The drawing under review shows one solid part. Ordinate dimensions are in mm from its lowest x, y, z. A direction names the side the tool comes from. Round coordinates to 2 decimals unless told otherwise and drop trailing zeros. Write each loop counter-clockwise with the first axis right and the second up, starting at its lowest first coordinate (ties: lowest second). Pieces come first, ordered by that corner, then holes.
Item 1: Add section A-A (z = 33). Give the boundary of the cut face in (x, y).
Item 2: Machinability: for the marked faces 1 and 2, which of the approach directions +Z, -Z, +X, -X, +Y, -Y give a long, thin tool a straight path to every point of the face, cutting with its end or side? Answer none if there is none.
Item 3: Add section C-C (x = 36.25). Give the boundary of the cut face in (y, z), plus the area to 3 significant figures.
Item 4: Clearance check with flat-ended pins moving along their axes: pin 1 Ø12 at (x, z) = (26, 10) entering from +Y; pin 2 Ø8 at (y, z) = (14, 29) entering from -X; pin 3 Ø2.5 at (x, z) = (33, 33) entering from +Y; pin 4 Ø8 at (y, z) = (15, 15.5) entering from -X. State where each tip first meets the part, or that it passes through.
Item 5: Add section B-B (x = 19). Give the boundary of the cut face in (y, z).
Item 6: Add section D-D (z = 19). Give the boundary of the cut face in (x, y), plus the area to 3 significant figures.
Item 7: To check wall thickness, follow L1, parallel to Z at x = 33, y = 0.4; L2, parallel to Z at x = 36.25, y = 0.8. State the ranges of each line that lie inside material, in increasing order.
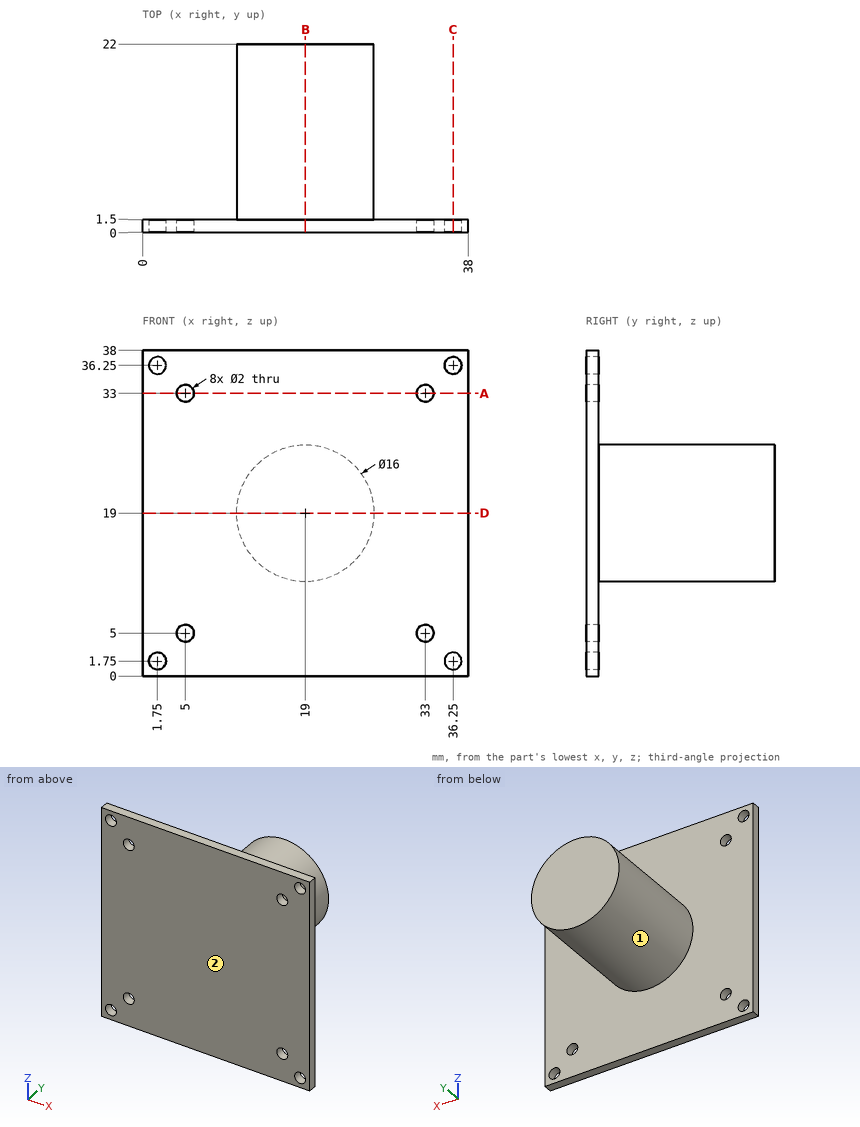
Numbers:
1. outline: (0, 0) - (4, 0) - (4, 1.5) - (0, 1.5) - close; (6, 0) - (32, 0) - (32, 1.5) - (6, 1.5) - close; (34, 0) - (38, 0) - (38, 1.5) - (34, 1.5) - close
2. face 1: +Y
2. face 2: +Z, -Z, +X, -X, -Y
3. outline: (0, 0) - (1.5, 0) - (1.5, 0.75) - (0, 0.75) - close; (0, 2.75) - (1.5, 2.75) - (1.5, 35.25) - (0, 35.25) - close; (0, 37.25) - (1.5, 37.25) - (1.5, 38) - (0, 38) - close
3. area: 51.0 mm2
4. pin 1: stops at y = 22
4. pin 2: stops at x = 13.71
4. pin 3: stops at y = 1.5
4. pin 4: stops at x = 11
5. outline: (0, 0) - (1.5, 0) - (1.5, 11) - (22, 11) - (22, 27) - (1.5, 27) - (1.5, 38) - (0, 38) - close
6. outline: (0, 0) - (38, 0) - (38, 1.5) - (27, 1.5) - (27, 22) - (11, 22) - (11, 1.5) - (0, 1.5) - close
6. area: 385 mm2
7. L1: z = 0 to 4, 6 to 32, 34 to 38
7. L2: z = 0 to 0.75, 2.75 to 35.25, 37.25 to 38
